```python
from build123d import *

# Parameters (mm, degrees)
SZKIC2_W                    = 22
SZKIC2_H                    = 120
DODANIE_WYCI_GNI_CIE1_DEPTH = 150
SZKIC3_R                    = 8
DODANIE_WYCI_GNI_CIE2_DEPTH = 15
SZYK_LINIOWY1_COUNT         = 2
SZYK_LINIOWY1_PITCH         = 40
SZYK_LINIOWY2_COUNT         = 2
SZYK_LINIOWY2_PITCH         = 135
SZYK_LINIOWY3_COUNT         = 2
SZYK_LINIOWY3_PITCH         = 95
SZKIC4_R                    = 8
DODANIE_WYCI_GNI_CIE3_DEPTH = 25
SZYK_LINIOWY4_COUNT         = 2
SZYK_LINIOWY4_PITCH         = 65


with BuildPart() as part:
    # Szkic2 → Dodanie-wyciągnięcie1 (new body)
    with BuildSketch(Plane(origin=(0, 0, 0), x_dir=(1, 0, 0), z_dir=(0, 1, 0))):
        Rectangle(SZKIC2_W, SZKIC2_H)
    extrude(amount=DODANIE_WYCI_GNI_CIE1_DEPTH)

    # Szkic3 → Dodanie-wyciągnięcie2 (add)
    with BuildSketch(Plane(origin=(0, 0, 0), x_dir=(1, 0, 0), z_dir=(0, 1, 0))):
        with BuildLine():
            Line((11, -16.864863098), (11, -60))
            ThreePointArc((11, -60), (18.004271641, -55.583996835), (26, -53.432431549))
            ThreePointArc((26, -53.432431549), (41, -38.432431549), (26, -23.432431549))
            ThreePointArc((26, -23.432431549), (18.004271641, -21.280866263), (11, -16.864863098))
        make_face()
        with Locations((26, -38.432431549)):
            Circle(SZKIC3_R, mode=Mode.SUBTRACT)
    dodanie_wyci_gni_cie2 = extrude(amount=DODANIE_WYCI_GNI_CIE2_DEPTH)

    # Szyk liniowy1: Dodanie-wyciągnięcie2 ×2
    with Locations(*[(0, i * SZYK_LINIOWY1_PITCH, 0) for i in range(1, SZYK_LINIOWY1_COUNT)]):
        add(dodanie_wyci_gni_cie2)

    # Szyk liniowy2: Dodanie-wyciągnięcie2 ×2
    with Locations(*[(0, i * SZYK_LINIOWY2_PITCH, 0) for i in range(1, SZYK_LINIOWY2_COUNT)]):
        add(dodanie_wyci_gni_cie2)

    # Szyk liniowy3: Dodanie-wyciągnięcie2 ×2
    with Locations(*[(0, i * SZYK_LINIOWY3_PITCH, 0) for i in range(1, SZYK_LINIOWY3_COUNT)]):
        add(dodanie_wyci_gni_cie2)

    # Szkic4 → Dodanie-wyciągnięcie3 (add)
    with BuildSketch(Plane(origin=(0, 30, 0), x_dir=(-1, 0, 0), z_dir=(0, -1, 0))):
        with BuildLine():
            Line((-11, 55.095776214), (-11, 8.216275777))
            ThreePointArc((-11, 8.216275777), (-17.948621334, 13.416118275), (-26, 16.656025995))
            ThreePointArc((-26, 16.656025995), (-41, 31.656025995), (-26, 46.656025995))
            ThreePointArc((-26, 46.656025995), (-17.948621334, 49.895933715), (-11, 55.095776214))
        make_face()
        with Locations((-26, 31.656025995)):
            Circle(SZKIC4_R, mode=Mode.SUBTRACT)
    dodanie_wyci_gni_cie3 = extrude(amount=-DODANIE_WYCI_GNI_CIE3_DEPTH)

    # Szyk liniowy4: Dodanie-wyciągnięcie3 ×2
    with Locations(*[(0, i * SZYK_LINIOWY4_PITCH, 0) for i in range(1, SZYK_LINIOWY4_COUNT)]):
        add(dodanie_wyci_gni_cie3)


solid = part.part
```
Could you check a few things on this model? Use its own coordinates, in mm. A direction names the side the tool comes from. Round coordinates to 2 decimals unless told otherwise and drop trailing zeros. Loops run counter-clockwise (first coordinate to the right, second up) from the corner with the lowest first, then second, coordinate; pieces in that order, holes last. Notation, with made-up numbers: (10, 26) - (38, 26) arc R7 ccw to (38, 35) - close; hole circle Ø3 at (54, -36). An arc over 180 degrees is marked (long way). Answer in a Markdown table with one row per item. Add a question column.
(1) If we section it at C-C (y = 26.5): Please give me the cut outline in (x, z), plus the area to 3 significant figures.
(2) If we section it at D-D (x = 22): State how many separate pieces and enclosed holes the cut face has, plus the area to 3 significant figures.
(3) I'm going to push flat-ended pins straight in: pin 1 (24 mm diameter, centred on x = 24.5, z = -26, fed in from -Y); pin 2 (21 mm diameter, centred on x = 26, z = -31.66, fed in from +Y); pin 3 (1 mm diameter, centred on x = 15, y = 115.5, fed in from -Z). Where does each tip first touch, or does it pass through?
(4) If we section it at A-A (y = 112): Please give me the cut outline in (x, z).
(5) If we mould it in two halves opening along X, with no side actions, what happens to faces 1 (the face through (20.1, 7.4, 33.03)), 2 (the face through (18.05, 107.32, -49.84)), 3 (the face through (19, 95, 43))? For each: pulls with the +X half, pulls with the -X half, needs draft (parallel to the pull), parting line crosses it, or undercut.
(6) If we section it at B-B (z = -4): Please give me the cut outline in (x, y), plus the area to 3 significant figures.
(7) I need wall thicknesses on line 1 along Z through (x, y) = (26, 101.75); line 2 along Y through (x, z) = (11.5, 37.5); line 3 along Y through (x, z) = (18, -49). Which ranges of each line are inside material? Lowest first, please.
(8) For faces 4 (the face through (19, 55, 43)), 5 (the face through (17.9, 142.4, 55.63)), 6 (the face through (18.111, 102.395, 21.327)), which set-ups out of +Z, -Z, +X, -X, +Y, -Y let a thin tool reach every point of the face, with its end or its side?
Model answer:
| question | item | result |
|---|---|---|
| 1 | outline | (-11, -60) - (11, -60) - (11, 60) - (-11, 60) - close |
| 1 | area | 2,640 mm² |
| 2 | separate pieces | 12 |
| 2 | enclosed holes | 0 |
| 2 | area | 2,000 mm² |
| 3 | pin 1 | stops at y = 30 |
| 3 | pin 2 | stops at y = 120 |
| 3 | pin 3 | stops at z = -52.13 |
| 4 | outline | (-11, -60) - (11, -60) - (11, -55.1) arc R33.49 cw to (26, -46.66) arc R15 ccw to (26, -16.66) arc R33.49 cw to (11, -8.22) - (11, 60) - (-11, 60) - close; hole circle Ø16 at (26, -31.66) |
| 5 | face 1 | undercut |
| 5 | face 2 | pulls with the +X half |
| 5 | face 3 | needs draft |
| 6 | outline | (-11, 0) - (11, 0) - (11, 150) - (-11, 150) - close |
| 6 | area | 3,300 mm² |
| 7 | line 1 | z = -46.66 to -39.66, -23.66 to -16.66, 23.43 to 30.43, 46.43 to 53.43 |
| 7 | line 2 | y = 0 to 15, 40 to 55, 95 to 110, 135 to 150 |
| 7 | line 3 | y = 30 to 55, 95 to 120 |
| 8 | face 4 | +Z, -Z, +X |
| 8 | face 5 | +Z, +X, +Y, -Y |
| 8 | face 6 | +X, +Y, -Y |
